Check sheet for the drawn part. Datum: minimum x, y, z corner. Units: mm. A direction names the side the tool comes from. Coordinates: 2 decimals unless noted, no trailing zeros. Write each loop counter-clockwise with the first axis right and the second up, starting at its lowest first coordinate (ties: lowest second). Pieces come first, ordered by that corner, then holes. Notation, with made-up numbers: M 42,36.25 L 50,36.25 A33 ccw 50,75.25 Z; hole C 27,-24.75 d4. An arc over 180 degrees is marked long. Answer in a Markdown table with one row per item.
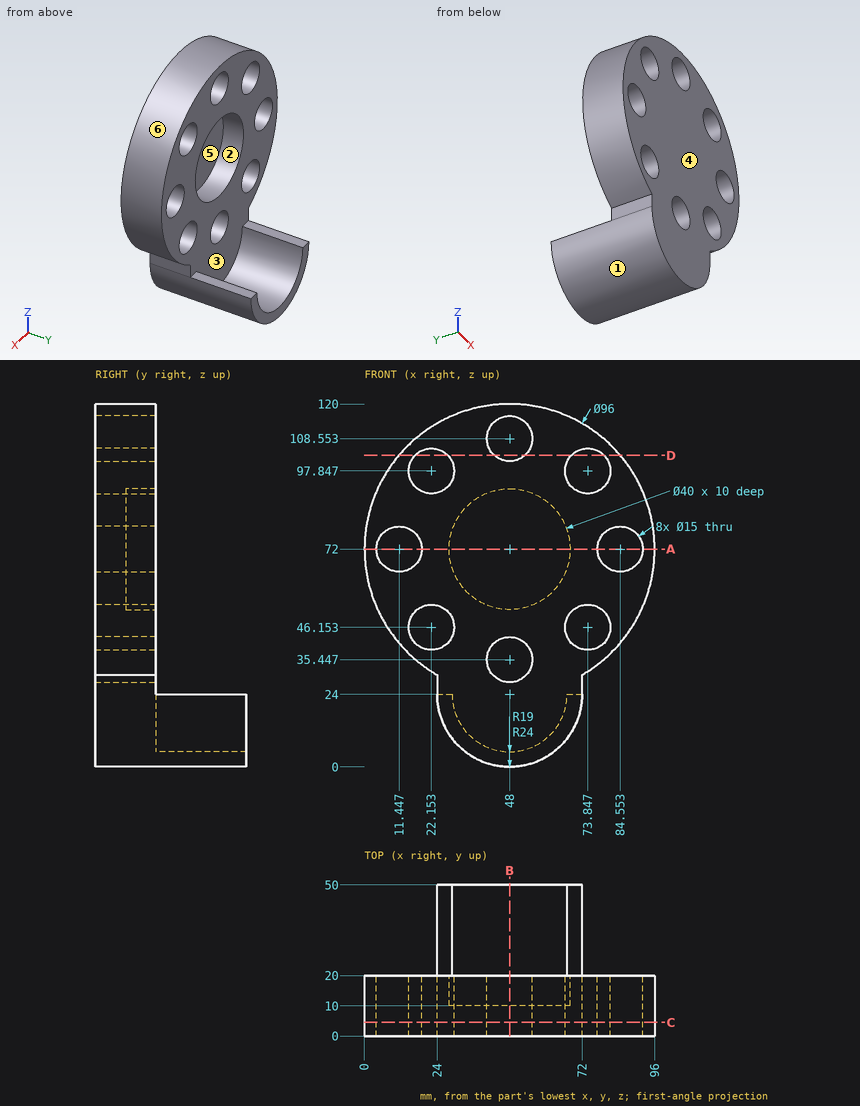
1) Sectioned sample at D-D (z = 103). Record the cut outline in (x, y).
Response values:
| item | result |
|---|---|
| outline | M 11.35,0 L 16.7,0 L 16.7,20 L 11.35,20 Z; M 27.6,0 L 42.96,0 L 42.96,20 L 27.6,20 Z; M 53.04,0 L 68.4,0 L 68.4,20 L 53.04,20 Z; M 79.3,0 L 84.65,0 L 84.65,20 L 79.3,20 Z |
2) Tool access check on the marked faces 1, 2 and 3. Record the directions out of +Z, -Z, +X, -X, +Y, -Y that give a thin tool (end or side, any length) a straight path to the whole face; none if there is none.
Response values:
| item | result |
|---|---|
| face 1 | -Z, +Y, -Y |
| face 2 | +Y |
| face 3 | +Z, +Y |
3) Depth check by flat-ended pin: pin 1 (7 mm diameter, centred on y = 14, z = 27, fed in from +X); pin 2 (24 mm diameter, centred on x = 22.15, z = 46.15, fed in from +Y); pin 3 (6 mm diameter, centred on x = 64.5, y = 19, fed in from -Z). Enter the tip coordinate at first touch or a pass-through.
Response values:
| item | result |
|---|---|
| pin 1 | stops at x = 72.12 |
| pin 2 | stops at y = 20 |
| pin 3 | stops at z = 4.16 |
4) Release check for a two-part mould opening along Z. For the marked faces 4, 5 and 6 record: +Z half, -Z half, draft (parallel to the pull), parting line (faces both ways), or undercut.
Response values:
| item | result |
|---|---|
| face 4 | draft |
| face 5 | undercut |
| face 6 | parting line |
5) Thickness scan on L1, parallel to X at y = 5.5, z = 72; L2, parallel to X at y = 3, z = 75; L3, parallel to Y at x = 49, z = 61. Record the ranges inside material, lowest first. Write a range as [from, to].
Response values:
| item | result |
|---|---|
| L1 | x = [0, 3.95], [18.95, 77.05], [92.05, 96] |
| L2 | x = [0.09, 4.57], [18.32, 77.68], [91.43, 95.91] |
| L3 | y = [0, 10] |
6) Sectioned sample at C-C (y = 4.5). Give the number of separate pieces and of enclosed holes in the cut face, then the cut area to 3 significant figures.
Response values:
| item | result |
|---|---|
| separate pieces | 1 |
| enclosed holes | 8 |
| area | 6,830 mm² |
7) Sectioned sample at A-A (z = 72). Record the cut outline in (x, y).
Response values:
| item | result |
|---|---|
| outline | M 0,0 L 3.95,0 L 3.95,20 L 0,20 Z; M 18.95,0 L 77.05,0 L 77.05,20 L 68,20 L 68,10 L 28,10 L 28,20 L 18.95,20 Z; M 92.05,0 L 96,0 L 96,20 L 92.05,20 Z |
8) Sectioned sample at B-B (x = 48). Record the cut outline in (y, z), then the cut area to 3 significant figures.
Response values:
| item | result |
|---|---|
| outline | M 0,0 L 50,0 L 50,5 L 20,5 L 20,27.95 L 0,27.95 Z; M 0,42.95 L 20,42.95 L 20,52 L 10,52 L 10,92 L 20,92 L 20,101.05 L 0,101.05 Z; M 0,116.05 L 20,116.05 L 20,120 L 0,120 Z |
| area | 1,550 mm² |
